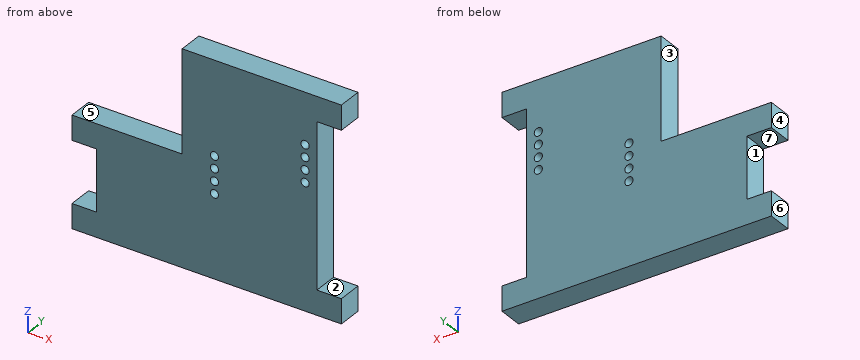
Autodesk Inventor part; units mm, degrees
ref_plane "YZ Plane" through (0, 0, 0) normal (1, 0, 0) x (0, 1, 0)
ref_plane "XZ Plane" through (0, 0, 0) normal (0, 1, 0) x (-1, 0, 0)
ref_plane "XY Plane" through (0, 0, 0) normal (0, 0, 1) x (1, 0, 0)
sketch "Sketch1" plane through (0, 0, 0) normal (0, 1, 0) x (-1, 0, 0)
  line L0 (0, 0) -> (60, 0)
  line L1 (66, 0) -> (66, 6)
  line L2 (66, 27) -> (60, 27)
  line L3 (0, 27) -> (0, 6) construction
  line L4 (66, 27) -> (60, 27)
  line L5 (60, 27) -> (60, 21) construction
  line L6 (60, 21) -> (66, 21)
  line L7 (66, 21) -> (66, 27)
  line L8 (66, 0) -> (60, 0)
  line L9 (60, 0) -> (60, 6) construction
  line L10 (60, 6) -> (66, 6)
  line L11 (66, 6) -> (66, 0)
  line L12 (66, 21) -> (66, 27)
  line L13 (60, 27) -> (6, 27)
  line L14 (60, 0) -> (66, 0)
  line L15 (66, 6) -> (66, 21) construction
  line L16 (60, 6) -> (60, 21)
  line L17 (0, 0) -> (6, 0)
  line L18 (6, 0) -> (6, 6) construction
  line L19 (6, 6) -> (0, 6)
  line L20 (0, 6) -> (0, 0)
  line L21 (6, 6) -> (6, 27)
  line L22 (6, 27) -> (0, 27) construction
  line L23 (0, 6) -> (0, 0)
  line L24 (6, 27) -> (39, 27)
  line L25 (39, 27) -> (39, 52)
  line L26 (39, 52) -> (6, 52)
  line L27 (6, 52) -> (0, 52)
  line L28 (0, 52) -> (0, 46)
  line L29 (0, 46) -> (6, 46)
  line L30 (6, 46) -> (6, 52) construction
  line L31 (6, 46) -> (6, 27)
  dimension "d0" = 66
  dimension "d1" = 27
  dimension "d2" = 6
  dimension "d3" = 6
  dimension "d4" = 6
  dimension "d5" = 6
  dimension "d6" = 6
  dimension "d7" = 6
  dimension "d10" = 33
  dimension "d11" = 25
  dimension "d12" = 6
  dimension "d13" = 6
extrude "Extrusion1" add sketch "Sketch1" along normal blind 6
sketch "Sketch2" plane through (0, 6, 0) normal (0, 1, 0) x (1, 0, 0)
  circle A0 centre (-8.9, -39.536) radius 1
  line L0 (0, -46) -> (-6, -46)
  line L1 (-6, -46) -> (-6, -6)
  circle A1 centre (-31.1, -29.236) radius 1
  circle A2 centre (-8.9, -36.536) radius 1
  circle A3 centre (-8.9, -33.536) radius 1
  circle A4 centre (-8.9, -30.536) radius 1
  circle A5 centre (-31.1, -26.236) radius 1
  circle A6 centre (-31.1, -23.236) radius 1
  circle A7 centre (-31.1, -20.236) radius 1
  point P0 (0, 0)
  dimension "d14" = 2
  dimension "d15" = 6.464
  dimension "d16" = 2.9
  dimension "d19" = 2
  dimension "d20" = 22.2
  dimension "d21" = 10.3
  dimension "d22" = 2
  dimension "d23" = 3
  dimension "d24" = 2
  dimension "d25" = 3
  dimension "d26" = 2
  dimension "d27" = 3
  dimension "d28" = 2
  dimension "d29" = 2
  dimension "d30" = 3
  dimension "d31" = 2
  dimension "d32" = 3
  dimension "d33" = 3
extrude "Extrusion2" cut sketch "Sketch2" against normal through all
properties part number "thumper-bumper-sidewall3-v2"
Check sheet for the modelled part. Datum: model origin and axes. Units: mm. Face numbers are marked on the shaded views. A direction names the side the tool comes from. Round coordinates to 2 decimals unless told otherwise and drop trailing zeros. Write each loop counter-clockwise with the first axis right and the second up, starting at its lowest first coordinate (ties: lowest second). Pieces come first, ordered by that corner, then holes. Notation, with made-up numbers: (0.5, 39.5) -> (42.5, 39.5) arc R21 cw to (42.5, 51.5) -> close; hole circle Ø1 at (-39, 88). An arc over 180 degrees is marked (long way). One line per question, with ' | ' between items. Start each with the question number.
1. Release check for a two-part mould opening along Z. For the marked faces 5, 6 and 7 record: +Z half, -Z half, draft (parallel to the pull), parting line (faces both ways), or undercut.
2. Sectioned sample at B-B, the plane y = 4.9. Count the separate pieces of the cut face and the enclosed holes in it, then the cut area to 3 significant figures.
3. Sectioned sample at D-D, the plane x = -56. Record the cut outline in (y, z), then the cut area to 3 significant figures.
4. Sectioned sample at C-C, the plane z = 7. Record the cut outline in (x, y).
5. Scan lines: line 1 along Z through (x, y) = (-31.1, 3.55); line 2 along Z through (x, y) = (-8.9, 1.6); line 3 along Z through (x, y) = (-63, 4.1). Record each from-to range of solid material in increasing order. Write a range as from..to.
6. Sectioned sample at A-A, the plane x = -31.1. Record the cut outline in (y, z), then the cut area to 3 significant figures.
7. Depth check by flat-ended pin: pin 1 (2.5 mm diameter, centred on x = -8.9, z = 33.536, fed in from -Y); pin 2 (1.8 mm diameter, centred on x = -31.1, z = 26.236, fed in from +Y); pin 3 (1 mm diameter, centred on y = 3.5, z = 33, fed in from -X); pin 4 (1.8 mm diameter, centred on x = -58.5, y = 2.5, fed in from +Z). Enter the tip coordinate at first touch or a pass-through.
8. Set-up check for the marked faces 1, 2, 3 and 4: record each of +Z, -Z, +X, -X, +Y, -Y from which the full face is reachable in a straight line by a thin tool's end or side.
Taken from the geometry:
1) face 5: +Z half | face 6: draft | face 7: undercut
2) separate pieces: 1 | enclosed holes: 8 | area: 2,400 mm^2
3) outline: (0, 0) -> (6, 0) -> (6, 27) -> (0, 27) -> close | area: 162 mm^2
4) outline: (-60, 0) -> (-6, 0) -> (-6, 6) -> (-60, 6) -> close
5) line 1: z = 0..19.24, 21.24..22.24, 24.24..25.24, 27.24..28.24, 30.24..52 | line 2: z = 0..29.54, 31.54..32.54, 34.54..35.54, 37.54..38.54, 40.54..52 | line 3: z = 0..6, 21..27
6) outline: (0, 0) -> (6, 0) -> (6, 19.24) -> (0, 19.24) -> close; (0, 21.24) -> (6, 21.24) -> (6, 22.24) -> (0, 22.24) -> close; (0, 24.24) -> (6, 24.24) -> (6, 25.24) -> (0, 25.24) -> close; (0, 27.24) -> (6, 27.24) -> (6, 28.24) -> (0, 28.24) -> close; (0, 30.24) -> (6, 30.24) -> (6, 52) -> (0, 52) -> close | area: 264 mm^2
7) pin 1: stops at y = 0 | pin 2: passes through | pin 3: stops at x = -39 | pin 4: stops at z = 27
8) face 1: -X, +Y, -Y | face 2: +X, +Y, -Y | face 3: +Z, -X, +Y, -Y | face 4: +Z, -Z, -X, +Y, -Y
